Build history of the part. All positions in model axes, mm. Give positions to 0.01 mm unless a question says otherwise; leave off trailing zeros. Write each loop counter-clockwise with the first axis right and the second up, starting at its lowest first coordinate (ties: lowest second). Pieces come first, ordered by that corner, then holes. Notation, with made-up numbers: M -17,41 L 26,41 A19 ccw 26,57 Z; hole C -32,-20.75 d3. An arc over 180 degrees is marked long. Return JSON: item names as keys, results as strings. Group by question number.
Q1. Band-saw the part on C-C, the plane x = 52. Give the cut face in (y, z).
Q2. Band-saw the part on A-A, the plane x = 18.25. Give the cut face in (y, z), then the cut area to 3 significant figures.
Q3. Wall check: probe 1 along X at (y, z) = (1.3, -43.5); probe 2 along X at (y, z) = (1.55, -11); probe 3 along X at (y, z) = (1.15, 0). Give the ranges that are in metal, low to high.
Q4. Band-saw the part on D-D, the plane z = -15. Give the cut face in (x, y).
Q5. Band-saw the part on B-B, the plane y = 1.1. Count the separate pieces of the cut face and the enclosed holes in it, then the cut area to 3 significant figures.
Q6. Flat gauge pins, fed straight in: pin 1 Ø3 at (x, y) = (4, 3) entering from +Z; pin 2 Ø1.5 at (y, z) = (1, 8) entering from +X. Where does each tip first touch, or does it go through?
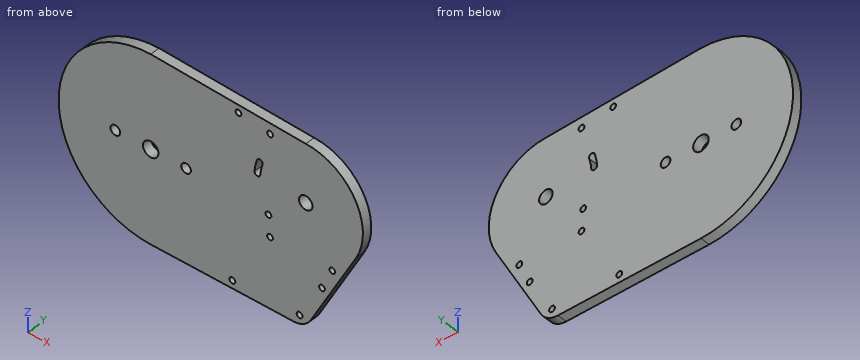
from build123d import *

# Parameters (mm, degrees)
SKETCH1_R           = 4
SKETCH1_R_2         = 1.5
SKETCH1_R_3         = 2.5
SKETCH1_R_4         = 3.5
BOSS_EXTRUDE1_DEPTH = 5


with BuildPart() as part:
    # Sketch1 → Boss-Extrude1 (new body)
    with BuildSketch(Plane(origin=(0, 0, 0), x_dir=(1, 0, 0), z_dir=(0, 1, 0))):
        with BuildLine():
            Line((0, -47.5), (80, -44.5))
            ThreePointArc((80, -44.5), (105.341650726, -30.101348895), (105.945295539, -0.961067014))
            Line((105.945295539, -0.961067014), (82.559049402, 42.258960334))
            ThreePointArc((82.559049402, 42.258960334), (78.883135286, 46.090390077), (73.764033965, 47.5))
            Line((73.764033965, 47.5), (0, 47.5))
            ThreePointArc((0, 47.5), (-47.5, 0), (0, -47.5))
        make_face()
        with Locations(Location((0, 0, 0), (0, 0, 270))):
            Circle(SKETCH1_R, mode=Mode.SUBTRACT)
        with Locations(Location((60.74263676, 0.942206906, 0), (0, 0, 270))):
            Circle(SKETCH1_R_2, mode=Mode.SUBTRACT)
        with Locations(Location((18.25, 0, 0), (0, 0, 270))):
            Circle(SKETCH1_R_3, mode=Mode.SUBTRACT)
        with Locations(Location((-18.25, 0, 0), (0, 0, 270))):
            Circle(SKETCH1_R_3, mode=Mode.SUBTRACT)
        with Locations(Location((80, -15, 0), (0, 0, 270))):
            Circle(SKETCH1_R_4, mode=Mode.SUBTRACT)
        with Locations(Location((76.835494757, 42.654234046, 0), (0, 0, 270))):
            Circle(SKETCH1_R_2, mode=Mode.SUBTRACT)
        with Locations(Location((88.354686129, 23.142870245, 0), (0, 0, 270))):
            Circle(SKETCH1_R_2, mode=Mode.SUBTRACT)
        with Locations(Location((42.137334928, 43.5, 0), (0, 0, 270))):
            Circle(SKETCH1_R_2, mode=Mode.SUBTRACT)
        with Locations(Location((45.293422434, -41.885064382, 0), (0, 0, 270))):
            Circle(SKETCH1_R_2, mode=Mode.SUBTRACT)
        with Locations(Location((61.591696316, 11.71100727, 0), (0, 0, 270))):
            Circle(SKETCH1_R_2, mode=Mode.SUBTRACT)
        with Locations(Location((93.688017257, 11.71100727, 0), (0, 0, 270))):
            Circle(SKETCH1_R_2, mode=Mode.SUBTRACT)
        with Locations(Location((61.591696316, -39.768646015, 0), (0, 0, 270))):
            Circle(SKETCH1_R_2, mode=Mode.SUBTRACT)
        with BuildLine():
            ThreePointArc((53.577406183, -17.023990113), (54.021018537, -20.229007757), (54.851917667, -23.356072939))
            ThreePointArc((54.851917667, -23.356072939), (56.748379286, -24.306564037), (57.698870384, -22.410102418))
            ThreePointArc((57.698870384, -22.410102418), (56.962035306, -19.637044615), (56.568643219, -16.794859157))
            ThreePointArc((56.568643219, -16.794859157), (54.958459223, -15.413806117), (53.577406183, -17.023990113))
        make_face(mode=Mode.SUBTRACT)
    extrude(amount=BOSS_EXTRUDE1_DEPTH)


solid = part.part
From the geometry:
{
 "1": {"outline": "M 0,-47.5 L 5,-47.5 L 5,45.55 L 0,45.55 Z"},
 "2": {"outline": "M 0,-47.5 L 5,-47.5 L 5,-2.5 L 0,-2.5 Z; M 0,2.5 L 5,2.5 L 5,46.82 L 0,46.82 Z", "area": "447 mm^2"},
 "3": {"probe 1": "x = -19.08 to 40.64, 43.64 to 75.6, 78.07 to 81.76", "probe 2": "x = -46.21 to 60.27, 62.91 to 92.37, 95.01 to 99.47", "probe 3": "x = -47.5 to -20.75, -15.75 to -4, 4 to 15.75, 20.75 to 59.58, 61.91 to 105.43"},
 "4": {"outline": "M -45.07,0 L 97.31,0 L 97.31,5 L -45.07,5 Z"},
 "5": {"separate pieces": "1", "enclosed holes": "13", "area": "12,500 mm^2"},
 "6": {"pin 1": "stops at z = 47.41", "pin 2": "stops at x = 108.83"}
}
